from build123d import *

# Parameters (mm, degrees)
F0_R     = 10
F0_R_2   = 3.1
F1_DEPTH = 5
F2_R     = 10
F2_R_2   = 3.1
F2_R_3   = 3
F3_DEPTH = 10
F4_DEPTH = 25


with BuildPart() as f1:
    # F0 (on Top) → F1 (new body)
    with BuildSketch(Plane.XY):
        Circle(F0_R)
        Circle(F0_R_2, mode=Mode.SUBTRACT)
    extrude(amount=F1_DEPTH)

    # F2 (on face) → F3 (join)
    with BuildSketch(Plane.XY.offset(5)):
        Circle(F2_R)
        Circle(F2_R_2, mode=Mode.SUBTRACT)
        Circle(F2_R_2)
        Circle(F2_R_3, mode=Mode.SUBTRACT)
    extrude(amount=F3_DEPTH)

    # F2 (on face) → F4 (join)
    with BuildSketch(Plane.XY.offset(5)):
        Circle(F2_R_3)
    extrude(amount=F4_DEPTH)


solid = f1.part
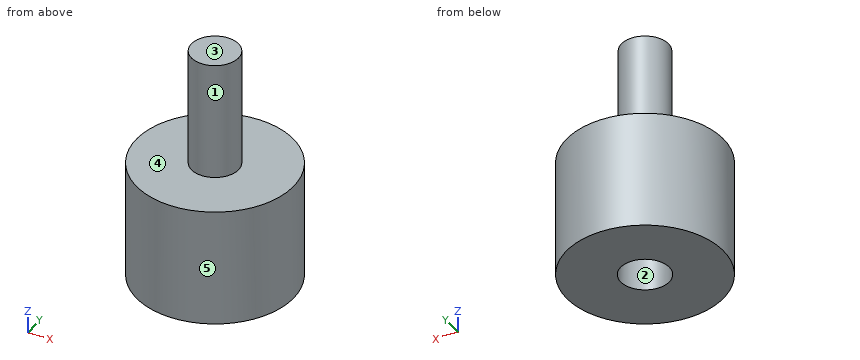
Model file for the job. Use its own axes, mm. Face numbers are marked on the shaded views. A direction names the side the tool comes from. Give positions to 0.01 mm unless a question says otherwise; leave off trailing zeros. Order: outer loops, then holes, each group sorted by start corner. A loop starts at its lowest first (then second) coordinate and runs counter-clockwise, first axis right, second up. Notation, with made-up numbers: (-11.5, 63) - (12.5, 63) arc R28 ccw to (12.5, 100) - close; hole circle Ø10 at (84.25, 47). An arc over 180 degrees is marked (long way). Write item = value, one per line. Start each with the question number.
1. Which spindle directions (+Z, -Z, +X, -X, +Y, -Y) get a long thin tool onto all of the face, cutting with end or side? Do the marked faces 4 and 5. Say none if no direction does.
2. Cut at D-D, the plane z = 25. List the corners of the cut face in (x, y), and give its area (3 significant figures).
3. Drop flat-ended pins along their axis: P1, Ø1, axis at x = 8, y = -7.5, coming from the -Z side; P2, Ø3, axis at x = 5.5, y = -2, coming from the +Z side; P3, Ø1, axis at y = 0.5, z = 24.5, coming from the -X side. Give the stop position or say it passes through.
4. Cut at C-C, the plane z = 14.5. List the corners of the cut face in (x, y), and give its area (3 significant figures).
5. Probe line 1 along Y through (x, z) = (0, 3.9); line 2 along Z through (x, y) = (4, -1.5); line 3 along X through (y, z) = (0.25, 8). List the from-to ranges inside material, lowest first.
6. Cut at A-A, the plane y = 0. List the corners of the cut face in (x, z), and give its area (3 significant figures).
7. Two-plate mould, pull along X, no slides. Class the marked faces 1, 2 and 3: pulls with the +X half, pulls with the -X half, needs draft (parallel to the pull), parting line crosses it, or undercut.
Taken from the geometry:
q1.face_4 = +Z
q1.face_5 = +Z, -Z
q2.outline = circle Ø6 at (0, 0)
q2.area = 28.3 mm²
q3.P1 = through
q3.P2 = 15
q3.P3 = -3
q4.outline = circle Ø20 at (0, 0)
q4.area = 314 mm²
q5.line_1 = -10 to -3.1, 3.1 to 10
q5.line_2 = 0 to 15
q5.line_3 = -10 to 10
q6.outline = (-10, 0) - (-3.1, 0) - (-3.1, 5) - (3.1, 5) - (3.1, 0) - (10, 0) - (10, 15) - (3, 15) - (3, 30) - (-3, 30) - (-3, 15) - (-10, 15) - close
q6.area = 359 mm²
q7.face_1 = parting line crosses it
q7.face_2 = undercut
q7.face_3 = needs draft
